For this review, take the finished solid that the model builds, in its own axes (mm). Face numbers are marked on the shaded views. Round coordinates to 2 decimals unless told otherwise and drop trailing zeros. Order: outer loops, then holes, each group sorted by start corner. A loop starts at its lowest first (then second) coordinate and runs counter-clockwise, first axis right, second up. Notation, with made-up numbers: M -0.75,60.25 L 45.25,60.25 A9 ccw 45.25,74.25 Z; hole C 52,-34 d9. An arc over 180 degrees is marked long. Answer as a JSON object with one key per item and string values.
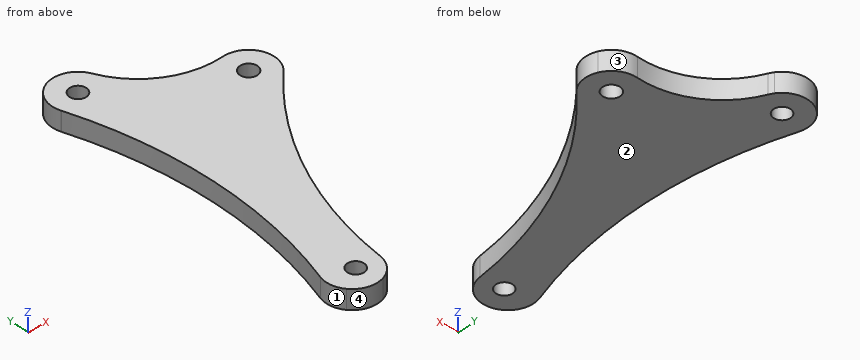
from build123d import *

# Parameters (mm, degrees)
SKETCH_1_R      = 1.3
SKETCH_1_R_2    = 1.35
EXTRUDE_1_DEPTH = 3


with BuildPart() as part:
    # 草图1 → 凸台-拉伸1 (new body)
    with BuildSketch(Plane.XY.offset(3)):
        with BuildLine():
            Line((-3.313115848, 16.021732214), (-3.311115848, 16.021732214))
            add(Edge.make_bspline(
                [(-3.311115848, 16.021732214), (-3.305738612, 16.005657169), (-3.30036747, 15.989580634), (-3.295002421, 15.973502613)],
                knots=[0, 0, 0, 0, 1, 1, 1, 1], degree=3))
            ThreePointArc((-3.295002421, 15.973502613), (0.247391506, -5.861355765), (-3.313115848, -27.693267786))
            ThreePointArc((-3.313115848, -27.693267786), (-3.460091003, -29.647679281), (-2.661550551, -31.43755613))
            ThreePointArc((-2.661550551, -31.43755613), (-0.621865458, -32.807647593), (1.833911351, -32.726246371))
            ThreePointArc((1.833911351, -32.726246371), (3.626794929, -31.434157055), (4.459911351, -29.387246371))
            ThreePointArc((4.459911351, -29.387246371), (9.614888081, -11.161248479), (20.542617881, 4.309546771))
            ThreePointArc((20.542617881, 4.309546771), (21.651368965, 6.44631062), (21.333617881, 8.832546771))
            ThreePointArc((21.333617881, 8.832546771), (19.703322731, 10.604311941), (17.351617881, 11.120546771))
            ThreePointArc((17.351617881, 11.120546771), (9.493211165, 12.888433489), (4.140617881, 18.907546771))
            ThreePointArc((4.140617881, 18.907546771), (3.968487676, 19.251416126), (3.76413819, 19.577170986))
            ThreePointArc((3.76413819, 19.577170986), (-1.314904342, 20.865715039), (-3.313115848, 16.021732214))
        make_face()
        with Locations(Location((0.853283407, -29.166236957, 0), (0, 0, 180))):
            Circle(SKETCH_1_R, mode=Mode.SUBTRACT)
        with Locations(Location((0.480884152, 17.291232214, 0), (0, 0, 180))):
            Circle(SKETCH_1_R, mode=Mode.SUBTRACT)
        with Locations(Location((17.711384152, 7.136232214, 0), (0, 0, 180))):
            Circle(SKETCH_1_R_2, mode=Mode.SUBTRACT)
    extrude(amount=-EXTRUDE_1_DEPTH)


solid = part.part
1) Mouldability with a two-part tool opening along Y and no side actions: class the marked faces 1, 2, 3 and 4 as +Y half, -Y half, draft (parallel to the pull), parting line (faces both ways), or undercut.
Geometry check:
{"face 1": "undercut", "face 2": "draft", "face 3": "+Y half", "face 4": "-Y half"}
2) For L1, parallel to Y at x = 18.5, z = 2.25; L2, parallel to Y at x = 16.5, z = 2; L3, parallel to X at y = -29, z = 0.85, list the stretches that pass through material, from the lowest coordinate up.
Geometry check:
{"L1": "y = 2.15 to 6.04, 8.23 to 11.06", "L2": "y = -0.2 to 6.54, 7.73 to 11.07", "L3": "x = -3.52 to -0.44, 2.14 to 4.5"}
3) Add section C-C on z = 0.85. State how many separate pieces and enclosed holes the cut face has, and give its area (3 significant figures).
Geometry check:
{"separate pieces": "1", "enclosed holes": "3", "area": "617 mm²"}
4) Insertion check: P1, Ø1, axis at x = 3.5, z = 2.5, coming from the +Y side. The pin has a flat end and moves straight along its axis. Give the tip position at first contact, or say it passes through.
Geometry check:
{"P1": "stops at y = 20.4"}
5) Add section D-D on x = 3.25. State the section outline as (y, z) points, and give its area (3 significant figures).
Geometry check:
{"outline": "M -31.85,0 L 20.18,0 L 20.18,3 L -31.85,3 Z", "area": "156 mm²"}
6) Add section B-B on y = -4. State the section outline as (x, z) points.
Geometry check:
{"outline": "M 0.22,0 L 13.7,0 L 13.7,3 L 0.22,3 Z"}
7) Add section A-A on x = 18. State the section outline as (y, z) points, and give its area (3 significant figures).
Geometry check:
{"outline": "M 1.59,0 L 5.82,0 L 5.82,3 L 1.59,3 Z; M 8.46,0 L 11.13,0 L 11.13,3 L 8.46,3 Z", "area": "20.7 mm²"}
